from build123d import *

# Parameters (mm, degrees)
EXTRUDE_THIN1_DEPTH = 914.4
FILLET1_R           = 1.905


with BuildPart() as part:
    # Sketch1 → Extrude-Thin1 (new body)
    with BuildSketch(Plane(origin=(0, 0, 0), x_dir=(0, 0, -1), z_dir=(1, 0, 0))):
        Polygon((-33.02, 12.7), (-45.72, 12.7), (-45.72, 0), (0, 0), (0, 81.28), (-45.72, 81.28), (-45.72, 68.58), (-33.02, 68.58), (-33.02, 63.5), (-50.8, 63.5), (-50.8, 86.36), (5.08, 86.36), (5.08, -5.08), (-50.8, -5.08), (-50.8, 17.78), (-33.02, 17.78), align=None)
    extrude(amount=EXTRUDE_THIN1_DEPTH)

    # Fillet1
    fillet1_edges = [part.edges().sort_by_distance(p)[0] for p in [
        (457.2, 12.7, 45.72),
        (457.2, 0, 45.72),
        (457.2, 0, 0),
        (457.2, 81.28, 0),
        (457.2, 81.28, 45.72),
        (457.2, 68.58, 45.72),
        (457.2, 68.58, 33.02),
        (457.2, 63.5, 33.02),
        (457.2, 63.5, 50.8),
        (457.2, 86.36, 50.8),
        (457.2, 86.36, -5.08),
        (457.2, -5.08, -5.08),
        (457.2, -5.08, 50.8),
        (457.2, 17.78, 50.8),
        (457.2, 17.78, 33.02),
        (457.2, 12.7, 33.02),
    ]]
    fillet(fillet1_edges, radius=FILLET1_R)


solid = part.part
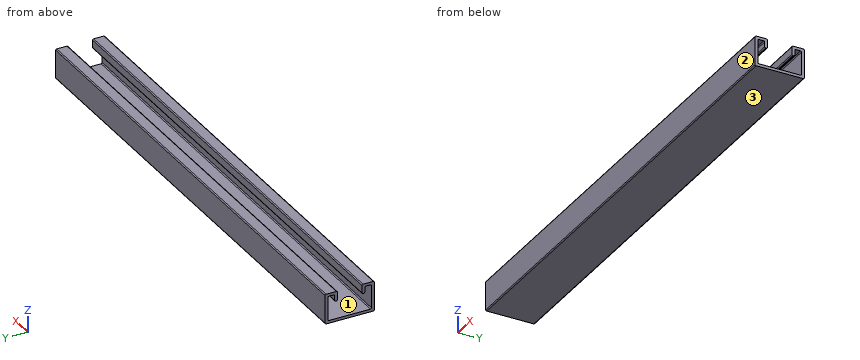
Input: part model. Units: mm. Frame: model coordinates. Face numbers are marked on the shaded views. Give positions to 0.01 mm unless a question says otherwise; leave off trailing zeros. Order: outer loops, then holes, each group sorted by start corner. A loop starts at its lowest first (then second) coordinate and runs counter-clockwise, first axis right, second up. Notation, with made-up numbers: (-8, 59) -> (20, 59) arc R22 ccw to (20, 71) -> close; hole circle Ø6 at (25, -10.5). An arc over 180 degrees is marked (long way). Use one line per item in the form item = value.
1) Mould query, pull axis Z, two halves, no side actions, for the marked faces 1, 2 and 3. Classes: pulls with the +Z half, pulls with the -Z half, needs draft (parallel to the pull), parting line crosses it, or undercut.
Response values:
face_1 = undercut
face_2 = needs draft
face_3 = pulls with the -Z half
2) Section A-A, the plane z = 12. Return loops of the section in (x, y).
Response values:
outline = (0, -5.08) -> (914.4, -5.08) -> (914.4, 0) -> (0, 0) -> close; (0, 81.28) -> (914.4, 81.28) -> (914.4, 86.36) -> (0, 86.36) -> close
3) Section C-C, the plane y = 46. Return loops of the section in (x, z).
Response values:
outline = (0, -5.08) -> (914.4, -5.08) -> (914.4, 0) -> (0, 0) -> close
4) First-contact query: pin 1 Ø23 at (x, y) = (509, 44) entering from +Z; pin 2 Ø1 at (y, z) = (12, 40.5) entering from +X. Flat tips, straight axial feed; report the tip coordinate or a pass-through.
Response values:
pin_1 = 0
pin_2 = through
5) Line query: probe 1 along Y at (x, z) = (787.5, 36.5); probe 2 along Y at (x, z) = (823.5, 7); probe 3 along Z at (x, y) = (485, 11.5). Output: solid intervals per line, ascending.
Response values:
probe_1 = -5.08 to 0, 12.7 to 17.78, 63.5 to 68.58, 81.28 to 86.36
probe_2 = -5.08 to 0, 81.28 to 86.36
probe_3 = -5.08 to 0, 45.58 to 50.8
